Part print with two shaded views. Sizes in mm from the minimum x, y, z corner. Give positions to 0.01 mm unless a question says otherwise; leave off trailing zeros. Write each loop counter-clockwise with the first axis right and the second up, starting at its lowest first coordinate (ties: lowest second). Pieces come first, ordered by that corner, then holes. Notation, with made-up numbers: (86, -24) - (131, -24) arc R10 ccw to (131, -18) - close; hole circle Ø11 at (87, 87.25). An arc over 180 degrees is marked (long way). Answer as a JSON object with one key per item and string values.
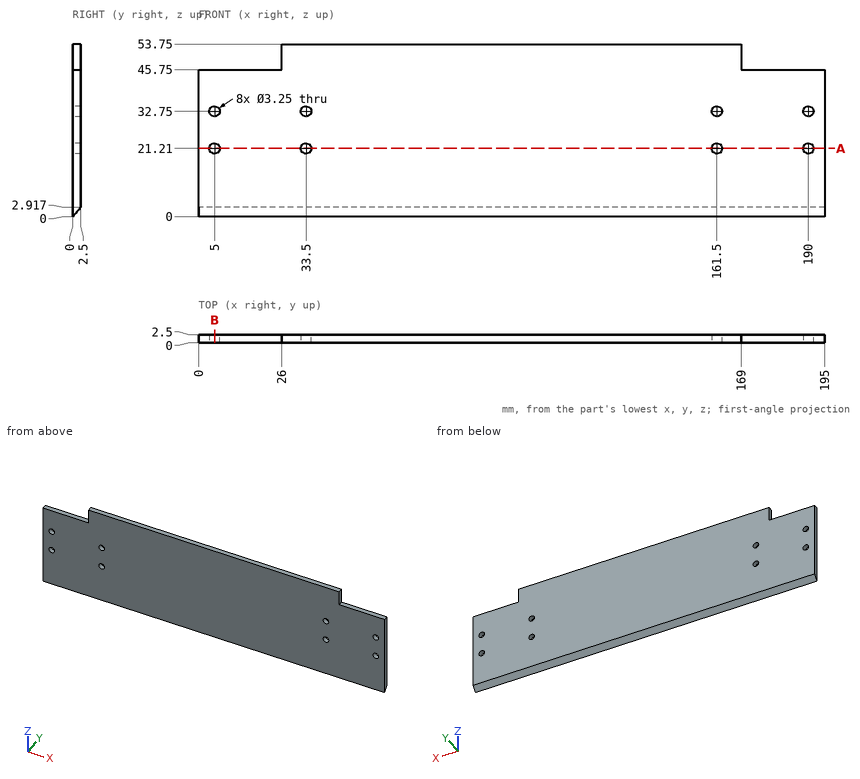
(1) Saw through at A-A, the plane z = 21.21. Give the cut face in (x, y) (3 decimals), and give its area (3 significant figures).
Answer key:
{"outline": "(0, 0) - (3.375, 0) - (3.375, 2.5) - (0, 2.5) - close; (6.625, 0) - (31.875, 0) - (31.875, 2.5) - (6.625, 2.5) - close; (35.125, 0) - (159.875, 0) - (159.875, 2.5) - (35.125, 2.5) - close; (163.125, 0) - (188.375, 0) - (188.375, 2.5) - (163.125, 2.5) - close; (191.625, 0) - (195, 0) - (195, 2.5) - (191.625, 2.5) - close", "area": "455 mm²"}
(2) Flat gauge pins, fed straight in: P1, Ø1.2, axis at x = 177, y = 1, coming from the +Z side; P2, Ø3, axis at x = 190, z = 32.75, coming from the +Y side; P3, Ø0.8, axis at y = 1.5, z = 49.5, coming from the -X side. Where does each tip first touch, or does it go through?
Answer key:
{"P1": "stops at z = 45.75", "P2": "passes through", "P3": "stops at x = 26"}
(3) Probe L1, parallel to X at y = 0.95, z = 32.75 (3 decimals); L2, parallel to Z at x = 118, y = 1.2; L3, parallel to Z at x = 136.5, y = 1.7. List the from-to ranges inside material, lowest first. Write a range as [from, to].
Answer key:
{"L1": "x = [0, 3.375], [6.625, 31.875], [35.125, 159.875], [163.125, 188.375], [191.625, 195]", "L2": "z = [1.4, 53.75]", "L3": "z = [1.98, 53.75]"}
(4) Saw through at B-B, the plane x = 5. State how many separate pieces and enclosed holes the cut face has.
Answer key:
{"separate pieces": "3", "enclosed holes": "0"}
